Geometry: final body of the model. Coordinates: model frame, mm. Face numbers are marked on the shaded views. Round coordinates to 2 decimals unless told otherwise and drop trailing zeros. Loops run counter-clockwise (first coordinate to the right, second up) from the corner with the lowest first, then second, coordinate; pieces in that order, holes last. Notation, with made-up numbers: M 72,24.25 L 78,24.25 A10 ccw 78,32.25 Z; hole C 1,-21.75 d6. An arc over 180 degrees is marked long. Return JSON: item names as keys, results as strings.
from build123d import *

# Parameters (mm, degrees)
BOSS_EXTRUDE6_DEPTH      = 2.9
SKETCH27_R               = 1.05
CUT_EXTRUDE12_DEPTH      = 3.9
SKETCH29_W               = 20
SKETCH29_H               = 4.356134153
BOSS_EXTRUDE8_DEPTH      = 11.5
BOSS_EXTRUDE8_DEPTH_BACK = 2.9
CUT_EXTRUDE13_DEPTH      = 15.4
FILLET1_R                = 2
SKETCH31_R               = 1
CUT_EXTRUDE14_DEPTH      = 4.656134153
CUT_EXTRUDE14_DEPTH_BACK = 24.656134153
CUT_EXTRUDE16_DEPTH      = 10
FILLET3_R                = 5
FILLET3_OF_MIRROR2_R     = 5


with BuildPart() as part:
    # Sketch26 → Boss-Extrude6 (new body)
    with BuildSketch(Plane(origin=(0, 0, 0), x_dir=(1, 0, 0), z_dir=(0, 1, 0))):
        with BuildLine():
            Line((-13.656134153, -7.7), (-13.656134153, 7.7))
            ThreePointArc((-13.656134153, 7.7), (0, 21.356134153), (13.656134153, 7.7))
            Line((13.656134153, 7.7), (13.656134153, -7.7))
            ThreePointArc((13.656134153, -7.7), (0, -21.356134153), (-13.656134153, -7.7))
        make_face()
        with BuildLine():
            Line((-8.5, 7.7), (-8.5, -7.7))
            ThreePointArc((-8.5, -7.7), (0, -16.2), (8.5, -7.7))
            Line((8.5, -7.7), (8.5, 7.7))
            ThreePointArc((8.5, 7.7), (0, 16.2), (-8.5, 7.7))
        make_face(mode=Mode.SUBTRACT)
    extrude(amount=BOSS_EXTRUDE6_DEPTH)

    # Sketch27 → Cut-Extrude12 (cut, through all)
    with BuildSketch(Plane(origin=(0, 2.9, 0), x_dir=(1, 0, 0), z_dir=(0, 1, 0))):
        with Locations((-8, 15)):
            Circle(SKETCH27_R)
        with Locations((8, 15)):
            Circle(SKETCH27_R)
        with Locations((8, -15)):
            Circle(SKETCH27_R)
        with Locations((-8, -15)):
            Circle(SKETCH27_R)
    extrude(amount=-CUT_EXTRUDE12_DEPTH, mode=Mode.SUBTRACT)

    # Sketch29 → Boss-Extrude8 (add, two sides)
    with BuildSketch(Plane(origin=(0, 2.9, 0), x_dir=(1, 0, 0), z_dir=(0, 1, 0))) as boss_extrude8_sk:
        with Locations((0, -19.178067076)):
            Rectangle(SKETCH29_W, SKETCH29_H)
    extrude(amount=BOSS_EXTRUDE8_DEPTH)
    extrude(boss_extrude8_sk.sketch, amount=-BOSS_EXTRUDE8_DEPTH_BACK)

    # Sketch30 → Cut-Extrude13 (cut, through all)
    with BuildSketch(Plane(origin=(0, 14.4, 0), x_dir=(1, 0, 0), z_dir=(0, 1, 0))):
        Polygon((-4, -21.356134153), (-6.515015226, -17), (6.515015226, -17), (4, -21.356134153), align=None)
    extrude(amount=-CUT_EXTRUDE13_DEPTH, mode=Mode.SUBTRACT)

    # Fillet1
    fillet1_edges = [part.edges().sort_by_distance(p)[0] for p in [
        (10, 7.2, 21.356134153),
        (10, 1.45, 17),
        (-10, 1.45, 17),
        (-10, 7.2, 21.356134153),
    ]]
    fillet(fillet1_edges, radius=FILLET1_R)

    # Sketch31 → Cut-Extrude14 (cut, two sides)
    with BuildSketch(Plane.ZY.offset(10)) as cut_extrude14_sk:
        with Locations((19, 7.9)):
            Circle(SKETCH31_R)
    extrude(amount=CUT_EXTRUDE14_DEPTH, mode=Mode.SUBTRACT)
    extrude(cut_extrude14_sk.sketch, amount=-CUT_EXTRUDE14_DEPTH_BACK, mode=Mode.SUBTRACT)

    # Sketch34 → Cut-Extrude16 (cut)
    with BuildSketch(Plane(origin=(0, 2.9, 0), x_dir=(1, 0, 0), z_dir=(0, 1, 0))):
        Polygon((-10, 9.72081528), (-6.01040764, 13.71040764), (-6.01040764, -13.71040764), (-10, -9.72081528), align=None)
    cut_extrude16 = extrude(amount=-CUT_EXTRUDE16_DEPTH, mode=Mode.SUBTRACT)

    # Fillet3
    fillet3_edges = [part.edges().sort_by_distance(p)[0] for p in [
        (-10, 1.45, 9.72081528),
        (-10, 1.45, -9.72081528),
    ]]
    fillet(fillet3_edges, radius=FILLET3_R)

    # Mirror2: Cut-Extrude16 across plane
    add(cut_extrude16.mirror(Plane(origin=(0, 0, 0), x_dir=(0, 0, 1), z_dir=(1, 0, 0))), mode=Mode.SUBTRACT)

    # Fillet3 of Mirror2
    fillet3_of_mirror2_edges = [part.edges().sort_by_distance(p)[0] for p in [
        (10, 1.45, 9.72081528),
        (10, 1.45, -9.72081528),
    ]]
    fillet(fillet3_of_mirror2_edges, radius=FILLET3_OF_MIRROR2_R)


solid = part.part
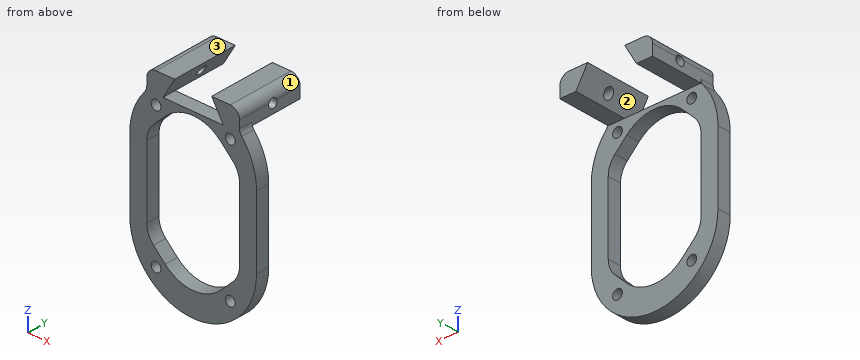
Q1. Section query B-B (y = 10). Output: boundary loops of the cut face in (x, z).
Determined:
{"outline": "M -10,17 L -6.52,17 L -4,21.36 L -8,21.36 A2 ccw -10,19.36 Z; M 4,21.36 L 6.52,17 L 10,17 L 10,19.36 A2 ccw 8,21.36 Z"}
Q2. Section query A-A (z = -4.5). Output: boundary loops of the cut face in (x, y), plus the area to 3 significant figures.
Determined:
{"outline": "M -13.66,0 L -10,0 L -10,2.9 L -13.66,2.9 Z; M 10,0 L 13.66,0 L 13.66,2.9 L 10,2.9 Z", "area": "21.2 mm^2"}
Q3. Pull-direction query (X, two-part tool) for the marked faces 1, 2 and 3; classes: pulls with the +X half, pulls with the -X half, needs draft (parallel to the pull), parting line crosses it, or undercut.
Determined:
{"face 1": "pulls with the +X half", "face 2": "undercut", "face 3": "needs draft"}
Q4. Material intervals for L1, parallel to X at y = 0.5, z = 6; L2, parallel to Z at x = 4.25, y = 1.25; L3, parallel to X at y = 0.65, z = 15, sorted ascending.
Determined:
{"L1": "x = -13.66 to -10, 10 to 13.66", "L2": "z = -20.68 to -15.06, 15.06 to 17, 20.92 to 21.36", "L3": "x = -11.54 to -9.05, -6.95 to -4.35, 4.35 to 6.95, 9.05 to 11.54"}
Q5. Section query D-D (y = 7.9). Output: boundary loops of the cut face in (x, z), plus the area to 3 significant figures.
Determined:
{"outline": "M -10,17 L -6.52,17 L -5.94,18 L -10,18 Z; M -9.89,20 L -4.78,20 L -4,21.36 L -8,21.36 A2 ccw Z; M 4,21.36 L 4.78,20 L 9.89,20 A2 ccw 8,21.36 Z; M 5.94,18 L 6.52,17 L 10,17 L 10,18 Z", "area": "21.1 mm^2"}
Q6. Section query C-C (x = 0.5). Output: boundary loops of the cut face in (y, z), plus the area to 3 significant figures.
Determined:
{"outline": "M 0,-21.35 L 2.9,-21.35 L 2.9,-16.19 L 0,-16.19 Z; M 0,16.19 L 2.9,16.19 L 2.9,17 L 0,17 Z", "area": "17.3 mm^2"}
Q7. Pin query (flat end, axial travel): pin 1 (2.5 mm diameter, centred on y = 7.9, z = 19, fed in from -X); pin 2 (2.5 mm diameter, centred on x = -2.5, y = 1.5, fed in from +Z); pin 3 (3.5 mm diameter, centred on x = -8, z = -15, fed in from +Y); pin 4 (1 mm diameter, centred on x = 11, y = 6, fed in from +Z). Return the tip coordinate at first contact, or that it passes through.
Determined:
{"pin 1": "stops at x = -10", "pin 2": "stops at z = 17", "pin 3": "stops at y = 2.9", "pin 4": "passes through"}
